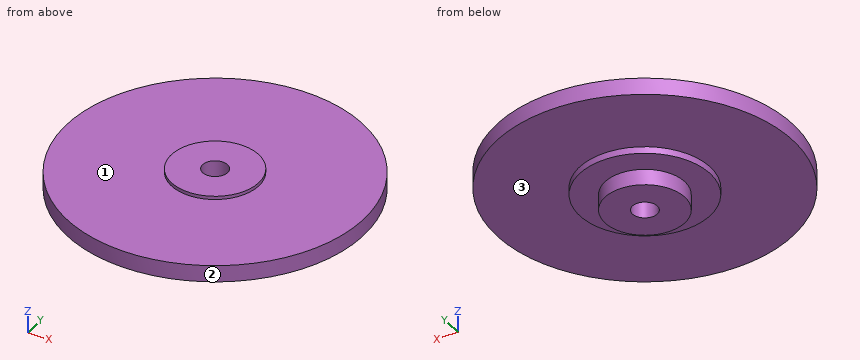
```python
from build123d import *

# Parameters (mm, degrees)
SKETCH_1_R          = 17.8
EXTRUDE_1_DEPTH     = 2
SKETCH_2_R          = 7.85
EXTRUDE_2_DEPTH     = 0.8
DRAFT_1_ANGLE       = 1
SKETCH_38_R         = 4.8
EXTRUDE_3_DEPTH     = 1.9
SKETCH_39_R         = 5.25
EXTRUDE_4_DEPTH     = 0.4
SKETCH_40_R         = 1.5
CUT_EXTRUDE_1_DEPTH = 10.4


with BuildPart() as part:
    # ｽｹｯﾁ1 → ﾎﾞｽ - 押し出し1 (new body)
    with BuildSketch(Plane.XY):
        Circle(SKETCH_1_R)
    extrude(amount=EXTRUDE_1_DEPTH)

    # ｽｹｯﾁ2 → ﾎﾞｽ - 押し出し2 (add)
    with BuildSketch(Plane(origin=(0, 0, 0), x_dir=(-1, 0, 0), z_dir=(0, 0, -1))):
        Circle(SKETCH_2_R)
    extrude(amount=EXTRUDE_2_DEPTH)

    # 抜き勾配1
    draft_1_faces = [part.faces().sort_by_distance(p)[0] for p in [
        (7.85, 0, -0.4),
    ]]
    draft(draft_1_faces, Plane(origin=(0, 0, -0.8), x_dir=(-1, 0, 0), z_dir=(0, 0, -1)), DRAFT_1_ANGLE)

    # ｽｹｯﾁ38 → ﾎﾞｽ - 押し出し3 (add)
    with BuildSketch(Plane(origin=(0, 0, -0.8), x_dir=(-1, 0, 0), z_dir=(0, 0, -1))):
        Circle(SKETCH_38_R)
    extrude(amount=EXTRUDE_3_DEPTH)

    # ｽｹｯﾁ39 → ﾎﾞｽ - 押し出し4 (add)
    with BuildSketch(Plane.XY.offset(2)):
        Circle(SKETCH_39_R)
    extrude(amount=EXTRUDE_4_DEPTH)

    # ｽｹｯﾁ40 → ｶｯﾄ - 押し出し1 (cut)
    with BuildSketch(Plane.XY.offset(2.4)):
        Circle(SKETCH_40_R)
    extrude(amount=-CUT_EXTRUDE_1_DEPTH, mode=Mode.SUBTRACT)


solid = part.part
```
The listing builds one solid part. Answer for the finished solid, in the listing's coordinates (mm). Face numbers are marked on the shaded views. A direction names the side the tool comes from. Give positions to 0.01 mm unless a question says otherwise; leave off trailing zeros. Loops run counter-clockwise (first coordinate to the right, second up) from the corner with the lowest first, then second, coordinate; pieces in that order, holes last. Notation, with made-up numbers: (24, 42.25) - (48, 42.25) arc R12 cw to (48, 63.25) - close; hole circle Ø1 at (74, 1). An arc over 180 degrees is marked (long way). Answer as CSV lines item,"result". Start each with the question number.
Item 1: For the marked faces 1, 2 and 3, determine the directions among +Z, -Z, +X, -X, +Y, -Y from which every point of the face is accessible in a straight line to the end or side of a thin tool.
Item 2: Find the intervals of material crossed by line 1 (Y direction, x = 0, z = 1.2); line 2 (Y direction, x = 0, z = -1.35); line 3 (Z direction, x = 4, y = -7), in increasing order. Write a range as from..to.
Item 3: A cutting plane is placed at A-A on x = 12. Determine the outline of the cut face in (y, z).
Item 4: A cutting plane is placed at B-B on y = -15. Determine the outline of the cut face in (x, z), then the cut area to 3 significant figures.
Item 5: Each of these flat-tipped pins is pushed along its axis until it touches: pin 1 (6 mm diameter, centred on x = 11.5, y = 3, fed in from -Z); pin 2 (12 mm diameter, centred on x = 5.5, y = 12.5, fed in from -Z). Where does it stop, or does it pass through?
Found:
1,face 1,"+Z"
1,face 2,"+Z, -Z"
1,face 3,"-Z"
2,line 1,"y = -17.8..-1.5, 1.5..17.8"
2,line 2,"y = -4.8..-1.5, 1.5..4.8"
2,line 3,"z = 0..2"
3,outline,"(-13.15, 0) - (13.15, 0) - (13.15, 2) - (-13.15, 2) - close"
4,outline,"(-9.58, 0) - (9.58, 0) - (9.58, 2) - (-9.58, 2) - close"
4,area,"38.3 mm^2"
5,pin 1,"stops at z = 0"
5,pin 2,"stops at z = -0.8"
